from build123d import *

# Parameters (mm, degrees)
ESQUISSE1_W             = 132
ESQUISSE1_H             = 60
BOSS_EXTRU_1_DEPTH      = 60
COQUE1_T                = -2
ESQUISSE2_W             = 15.270123606
ESQUISSE2_H             = 15.006197758
ENL_V_MAT_EXTRU_3_DEPTH = 150
ESQUISSE3_W             = 15.1141578
ESQUISSE3_H             = 15.542141472
ENL_V_MAT_EXTRU_4_DEPTH = 150


with BuildPart() as part:
    # Esquisse1 → Boss.-Extru.1 (new body)
    with BuildSketch(Plane(origin=(0, 0, 0), x_dir=(1, 0, 0), z_dir=(0, 1, 0))):
        with Locations((66, 30)):
            Rectangle(ESQUISSE1_W, ESQUISSE1_H)
    extrude(amount=BOSS_EXTRU_1_DEPTH)

    # Coque1
    coque1_openings = [part.faces().sort_by_distance(p)[0] for p in [
        (66, 60, -30),
    ]]
    offset(amount=COQUE1_T, openings=coque1_openings, kind=Kind.INTERSECTION)

    # Esquisse2 → Enlèv. mat.-Extru.3 (cut)
    with BuildSketch(Plane(origin=(2, 0, 0), x_dir=(0, 0, -1), z_dir=(1, 0, 0))):
        with Locations((45.027247918, 9.503098879)):
            Rectangle(ESQUISSE2_W, ESQUISSE2_H)
    extrude(amount=-ENL_V_MAT_EXTRU_3_DEPTH, mode=Mode.SUBTRACT)

    # Esquisse3 → Enlèv. mat.-Extru.4 (cut)
    with BuildSketch(Plane.ZY.offset(-130)):
        with Locations((-14.874699742, 9.771070736)):
            Rectangle(ESQUISSE3_W, ESQUISSE3_H)
    extrude(amount=-ENL_V_MAT_EXTRU_4_DEPTH, mode=Mode.SUBTRACT)


solid = part.part
Source: CAD feature listing. Evaluate the final solid. Frame: model axes, mm. A direction names the side the tool comes from. Round coordinates to 2 decimals unless told otherwise and drop trailing zeros. Loops run counter-clockwise (first coordinate to the right, second up) from the corner with the lowest first, then second, coordinate; pieces in that order, holes last. Notation, with made-up numbers: (58, -12.5) - (109, -12.5) arc R21 ccw to (109, 1.5) - close; hole circle Ø4 at (13, 60). An arc over 180 degrees is marked (long way). Write item = value, one per line. Start each with the question number.
(1) Pull-direction query (Z, two-part tool) for faces 1 (the face through (65, 30, 0)), 2 (the face through (0, 30, -30)), 3 (the face through (130, 31, -30)); classes: +Z half, -Z half, draft (parallel to the pull), parting line (faces both ways), or undercut.
(2) Ray query, line 1 along Z through (x, y) = (16, 55); line 2 along X through (y, z) = (13.5, -34.5); line 3 along X through (y, z) = (4, -50.5). Return the intervals inside material, ascending. Write a range as from..to.
(3) Section query B-B, the plane z = -48. Output: boundary loops of the cut face in (x, y), plus the area to 3 significant figures.
(4) Section query C-C, the plane y = 54.5. Output: boundary loops of the cut face in (x, z), plus the area to 3 significant figures.
(5) Section query A-A, the plane y = 11. Output: boundary loops of the cut face in (x, z), plus the area to 3 significant figures.
(6) Section query D-D, the plane x = 62.5. Output: boundary loops of the cut face in (y, z).
(7) Pin query (flat end, axial travel): pin 1 (17 mm diameter, centred on x = 53, z = -32.5, fed in from +Y). Return the tip coordinate at first contact, or that it passes through.
(8) Set-up query: faces 4 (the face through (65, 31, -58)), 5 (the face through (65, 30, -60)). Return all of +Z, -Z, +X, -X, +Y, -Y with unobstructed straight access to the full face (end or side cutting, diameter ignored); none if empty.
Conclusion:
q1.face_1 = +Z half
q1.face_2 = draft
q1.face_3 = undercut
q2.line_1 = -60..-58, -2..0
q2.line_2 = 0..2, 130..132
q2.line_3 = 130..132
q3.outline = (0, 0) - (132, 0) - (132, 60) - (130, 60) - (130, 2) - (0, 2) - close; (0, 17.01) - (2, 17.01) - (2, 60) - (0, 60) - close
q3.area = 466 mm2
q4.outline = (0, -60) - (132, -60) - (132, 0) - (0, 0) - close; hole (2, -58) - (130, -58) - (130, -2) - (2, -2) - close
q4.area = 752 mm2
q5.outline = (0, -60) - (132, -60) - (132, -22.43) - (130, -22.43) - (130, -58) - (2, -58) - (2, -52.66) - (0, -52.66) - close; (0, -37.39) - (2, -37.39) - (2, -2) - (130, -2) - (130, -7.32) - (132, -7.32) - (132, 0) - (0, 0) - close
q5.area = 691 mm2
q6.outline = (0, -60) - (60, -60) - (60, -58) - (2, -58) - (2, -2) - (60, -2) - (60, 0) - (0, 0) - close
q7.pin_1 = 2
q8.face_4 = +Y
q8.face_5 = -Z, +X, -X, +Y, -Y
